Build history of the part. All positions in model axes, mm. Face numbers are marked on the shaded views. Give positions to 0.01 mm unless a question says otherwise; leave off trailing zeros. Loops run counter-clockwise (first coordinate to the right, second up) from the corner with the lowest first, then second, coordinate; pieces in that order, holes last. Notation, with made-up numbers: M 0.25,86 L 37.25,86 A22 ccw 37.25,112 Z; hole C 78.5,79 d9. An arc over 180 degrees is marked long. Answer as a JSON object with one key per item and string values. Group by question number.
1. Slice it at D-D (x = 0). List the corners of the cut face in (y, z), then the cut area to 3 significant figures.
2. Drill centre lines: line 1 along X through (y, z) = (181, 26); line 2 along X through (y, z) = (161, 59); line 3 along Z through (x, y) = (60, 176.5). Where is each one in solid material? Low to high. Write a range as [from, to].
3. Slice it at B-B (y = 78). List the corners of the cut face in (x, z), then the cut area to 3 significant figures.
4. Slice it at A-A (z = 50). List the corners of the cut face in (x, y), then the cut area to 3 significant figures.
5. Slice it at C-C (z = 11). List the corners of the cut face in (x, y).
6. Mould opens along Z. For the marked faces 1 and 2 say: released by +Z, released by -Z, zero draft, split by the parting line, or undercut.
7. Drop flat-ended pins along their axis: pin 1 Ø4 at (y, z) = (120.5, 64) entering from -X; pin 2 Ø2 at (y, z) = (65.5, 42) entering from -X; pin 3 Ø4 at (y, z) = (95.5, 33.5) entering from -X. Give the stop position or say it passes through.
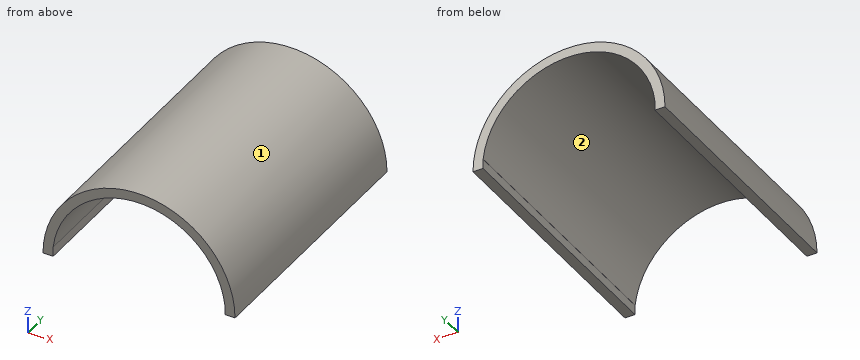
from build123d import *

# Parameters (mm, degrees)
BOSS_EXTRUDE1_DEPTH = 203.2
CUT_EXTRUDE1_DEPTH  = 203.2
SKETCH3_W           = 136.421155183
SKETCH3_H           = 7.62
CUT_EXTRUDE2_DEPTH  = 203.2


with BuildPart() as part:
    # Sketch1 → Boss-Extrude1 (new body)
    with BuildSketch(Plane(origin=(0, 0, 0), x_dir=(1, 0, 0), z_dir=(0, 1, 0))):
        with BuildLine():
            Line((-76.2, 0), (76.2, 0))
            ThreePointArc((76.2, 0), (0, -76.2), (-76.2, 0))
        make_face()
    extrude(amount=BOSS_EXTRUDE1_DEPTH)

    # Sketch2 → Cut-Extrude1 (cut)
    with BuildSketch(Plane(origin=(0, 203.2, 0), x_dir=(1, 0, 0), z_dir=(0, 1, 0))):
        with BuildLine():
            Line((68.155351954, -7.62), (-68.155351954, -7.62))
            ThreePointArc((-68.155351954, -7.62), (0, -68.58), (68.155351954, -7.62))
        make_face()
    extrude(amount=-CUT_EXTRUDE1_DEPTH, mode=Mode.SUBTRACT)

    # Sketch3 → Cut-Extrude2 (cut)
    with BuildSketch(Plane(origin=(0, 203.2, 0), x_dir=(1, 0, 0), z_dir=(0, 1, 0))):
        with Locations((0.055225637, -3.81)):
            Rectangle(SKETCH3_W, SKETCH3_H)
    extrude(amount=-CUT_EXTRUDE2_DEPTH, mode=Mode.SUBTRACT)


solid = part.part
Established:
{
 "1": {"outline": "M 0,68.58 L 203.2,68.58 L 203.2,76.2 L 0,76.2 Z", "area": "1,550 mm^2"},
 "2": {"line 1": "x = [-71.63, -63.46], [63.46, 71.63]", "line 2": "x = [-48.22, -34.96], [34.96, 48.22]", "line 3": "z = [33.21, 46.97]"},
 "3": {"outline": "M -76.2,0 L -68.16,0 L -68.16,7.62 A68.58 cw 68.16,7.62 L 68.27,7.62 L 68.27,0 L 76.2,0 A76.2 ccw Z", "area": "1,740 mm^2"},
 "4": {"outline": "M -57.5,0 L -46.94,0 L -46.94,203.2 L -57.5,203.2 Z; M 46.94,0 L 57.5,0 L 57.5,203.2 L 46.94,203.2 Z", "area": "4,290 mm^2"},
 "5": {"outline": "M -75.4,0 L -67.69,0 L -67.69,203.2 L -75.4,203.2 Z; M 67.69,0 L 75.4,0 L 75.4,203.2 L 67.69,203.2 Z"},
 "6": {"face 1": "released by +Z", "face 2": "released by -Z"},
 "7": {"pin 1": "stops at x = -44.3", "pin 2": "stops at x = -64.23", "pin 3": "stops at x = -69.38"}
}
